Autodesk Inventor part; units mm, degrees
ref_plane "YZ Plane" through (0, 0, 0) normal (1, 0, 0) x (0, 1, 0)
ref_plane "XZ Plane" through (0, 0, 0) normal (0, 1, 0) x (-1, 0, 0)
ref_plane "XY Plane" through (0, 0, 0) normal (0, 0, 1) x (1, 0, 0)
sketch "Sketch1" plane through (0, 0, 0) normal (0, 0, 1) x (1, 0, 0)
  line L0 (-5.91, 5.4476) -> (654.49, 5.4476)
  line L1 (654.49, 5.4476) -> (654.49, -19.9524)
  line L2 (654.49, -19.9524) -> (-5.91, -19.9524)
  line L3 (-5.91, -19.9524) -> (-5.91, 5.4476)
  point P0 (0, 0)
  dimension "d0" = 660.4
  dimension "d1" = 25.4
extrude "Extrusion1" add sketch "Sketch1" along normal blind 25.4
sketch "Sketch2" plane through (0, 0, 25.4) normal (0, 0, 1) x (1, 0, 0)
  circle A0 centre (6.79, -7.2524) radius 1.9685
  line L0 (-5.91, 5.4476) -> (-5.91, -19.9524)
  line L1 (-5.91, -19.9524) -> (654.49, -19.9524)
  circle A1 centre (32.19, -7.2524) radius 1.9685
  circle A2 centre (57.59, -7.2524) radius 1.9685
  circle A3 centre (82.99, -7.2524) radius 1.9685
  circle A4 centre (108.39, -7.2524) radius 1.9685
  circle A5 centre (133.79, -7.2524) radius 1.9685
  circle A6 centre (159.19, -7.2524) radius 1.9685
  circle A7 centre (184.59, -7.2524) radius 1.9685
  circle A8 centre (209.99, -7.2524) radius 1.9685
  circle A9 centre (235.39, -7.2524) radius 1.9685
  circle A10 centre (260.79, -7.2524) radius 1.9685
  circle A11 centre (286.19, -7.2524) radius 1.9685
  circle A12 centre (311.59, -7.2524) radius 1.9685
  circle A13 centre (336.99, -7.2524) radius 1.9685
  circle A14 centre (362.39, -7.2524) radius 1.9685
  circle A15 centre (387.79, -7.2524) radius 1.9685
  circle A16 centre (413.19, -7.2524) radius 1.9685
  circle A17 centre (438.59, -7.2524) radius 1.9685
  circle A18 centre (463.99, -7.2524) radius 1.9685
  circle A19 centre (489.39, -7.2524) radius 1.9685
  circle A20 centre (514.79, -7.2524) radius 1.9685
  circle A21 centre (540.19, -7.2524) radius 1.9685
  circle A22 centre (565.59, -7.2524) radius 1.9685
  circle A23 centre (590.99, -7.2524) radius 1.9685
  circle A24 centre (616.39, -7.2524) radius 1.9685
  circle A25 centre (641.79, -7.2524) radius 1.9685
  point P0 (0, 0)
  dimension "d4" = 3.937
  dimension "d5" = 12.7
  dimension "d6" = 12.7
  dimension "d9" = 25.4
  dimension "d16" = 25.4
extrude "Extrusion2" cut sketch "Sketch2" against normal blind 25.4
sketch "Sketch3" plane through (-5.91, -19.9524, 0) normal (-1, 0, 0) x (0, 0, 1)
  line L0 (3.175, 22.225) -> (22.225, 22.225)
  line L1 (22.225, 22.225) -> (22.225, 3.175)
  line L2 (22.225, 3.175) -> (3.175, 3.175)
  line L3 (3.175, 3.175) -> (3.175, 22.225)
  line L4 (0, 25.4) -> (25.4, 25.4)
  line L5 (0, 0) -> (0, 25.4)
  line L6 (0, 0) -> (25.4, 0)
  line L7 (25.4, 25.4) -> (25.4, 0)
  point P0 (0, 19.9524)
  dimension "d23" = 3.175
  dimension "d24" = 3.175
  dimension "d25" = 3.175
  dimension "d26" = 3.175
sketch "Sketch4" plane through (-5.91, 5.4476, 0) normal (0, 1, 0) x (1, 0, 0)
  circle A0 centre (12.7, -12.7) radius 1.9685
  line L0 (0, 0) -> (0, -25.4)
  line L1 (660.4, -25.4) -> (0, -25.4)
  circle A1 centre (38.1, -12.7) radius 1.9685
  circle A2 centre (63.5, -12.7) radius 1.9685
  circle A3 centre (88.9, -12.7) radius 1.9685
  circle A4 centre (114.3, -12.7) radius 1.9685
  circle A5 centre (139.7, -12.7) radius 1.9685
  circle A6 centre (165.1, -12.7) radius 1.9685
  circle A7 centre (190.5, -12.7) radius 1.9685
  circle A8 centre (215.9, -12.7) radius 1.9685
  circle A9 centre (241.3, -12.7) radius 1.9685
  circle A10 centre (266.7, -12.7) radius 1.9685
  circle A11 centre (292.1, -12.7) radius 1.9685
  circle A12 centre (317.5, -12.7) radius 1.9685
  circle A13 centre (342.9, -12.7) radius 1.9685
  circle A14 centre (368.3, -12.7) radius 1.9685
  circle A15 centre (393.7, -12.7) radius 1.9685
  circle A16 centre (419.1, -12.7) radius 1.9685
  circle A17 centre (444.5, -12.7) radius 1.9685
  circle A18 centre (469.9, -12.7) radius 1.9685
  circle A19 centre (495.3, -12.7) radius 1.9685
  circle A20 centre (520.7, -12.7) radius 1.9685
  circle A21 centre (546.1, -12.7) radius 1.9685
  circle A22 centre (571.5, -12.7) radius 1.9685
  circle A23 centre (596.9, -12.7) radius 1.9685
  circle A24 centre (622.3, -12.7) radius 1.9685
  circle A25 centre (647.7, -12.7) radius 1.9685
  point P0 (5.91, 0)
  dimension "d27" = 3.937
  dimension "d28" = 12.7
  dimension "d29" = 12.7
  dimension "d32" = 25.4
extrude "Extrusion3" cut sketch "Sketch4" against normal blind 25.4
extrude "Extrusion4" cut sketch "Sketch3" against normal blind 660.4 contours L0 L1 L2 L3
sketch "Sketch5" plane through (654.49, -19.9524, 0) normal (1, 0, 0) x (0, 0, -1)
  line L0 (-25.4, 25.4) -> (-25.4, 0)
  line L1 (-25.4, 25.4) -> (0, 25.4)
  line L2 (0, 25.4) -> (0, 0)
  line L3 (0, 0) -> (-25.4, 0)
  line L4 (-25.4, 0) -> (-25.4, 25.4)
  point P0 (0, 19.9524)
extrude "Extrusion5" cut sketch "Sketch5" against normal blind 381
properties part number "real numbah 9"
Design review of the part built by this model. Coordinates are the model's own, in mm. A direction names the side the tool comes from. Coordinates: 2 decimals unless noted, no trailing zeros. Write each loop counter-clockwise with the first axis right and the second up, starting at its lowest first coordinate (ties: lowest second). Pieces come first, ordered by that corner, then holes.
1) Machinability: for faces 4 (the flat face through (136, -19.952, 15)), 5 (the flat face through (132, -5, 3.175)), which of the approach directions +Z, -Z, +X, -X, +Y, -Y give a long, thin tool a straight path to every point of the face, cutting with its end or side? Answer none if there is none.
2) Add section C-C (y = -14.25). Write out the cut boundary in (x, z) (3 decimals), plus the area to 3 significant figures.
3) To check wall thickness, follow L1, parallel to Z at x = 235.39, y = 3.5; L2, parallel to Z at x = 237, y = -1.75 (3 decimals); L3, parallel to Y at x = 138.5, z = 12. State the ranges of each line that lie inside material, in increasing order.
4) Add section B-B (x = 245.5). Write out the cut boundary in (y, z) (3 decimals), plus the area to 3 significant figures.
5) Mouldability with a two-part tool opening along Y and no side actions: class faces 1 (the flat face through (132, -4, 25.4)), 2 (the flat face through (132, 5.448, 15)), 3 (the flat face through (132, -5, 22.225)) as +Y half, -Y half, draft (parallel to the pull), parting line (faces both ways), or undercut.
6) Add section A-A (z = 7.25). Write out the cut boundary in (x, y), plus the area to 3 significant figures.
7) Insertion check: pin 1 (3.5 mm diameter, centred on x = 260.79, y = -7.25, fed in from +Z); pin 2 (4.5 mm diameter, centred on x = 32.19, z = 12.7, fed in from +Y). Each pin has a flat end and moves straight along its axis. Give the tip position at first contact, or say it passes through.
Check result:
1. face 4: +Z, -Z, +X, -X, -Y
1. face 5: +X, -X
2. outline: (-5.91, 0) - (273.49, 0) - (273.49, 3.175) - (-5.91, 3.175) - close; (-5.91, 22.225) - (273.49, 22.225) - (273.49, 25.4) - (-5.91, 25.4) - close
2. area: 1,770 mm2
3. L1: z = 0 to 10.73, 14.67 to 25.4
3. L2: z = 0 to 3.175, 22.225 to 25.4
3. L3: y = -19.95 to -16.78, 2.27 to 5.45
4. outline: (-19.952, 0) - (5.448, 0) - (5.448, 25.4) - (-19.952, 25.4) - close; hole (-16.777, 3.175) - (2.273, 3.175) - (2.273, 22.225) - (-16.777, 22.225) - close
4. area: 282 mm2
5. face 1: draft
5. face 2: +Y half
5. face 3: undercut
6. outline: (-5.91, -19.95) - (273.49, -19.95) - (273.49, -16.78) - (-5.91, -16.78) - close; (-5.91, 2.27) - (273.49, 2.27) - (273.49, 5.45) - (-5.91, 5.45) - close
6. area: 1,770 mm2
7. pin 1: passes through
7. pin 2: stops at y = 5.45
